```python
from build123d import *

# Parameters (mm, degrees)
SKETCH1_R           = 2
SKETCH1_R_2         = 2.7
SKETCH1_R_3         = 6.5
BOSS_EXTRUDE1_DEPTH = 2
SKETCH1_3_R         = 4.5
SKETCH1_3_R_2       = 3.5
SKETCH1_3_R_3       = 2
BOSS_EXTRUDE2_DEPTH = 26
CUT_EXTRUDE1_START  = -26
SKETCH1_4_R         = 4.5
SKETCH1_4_R_2       = 3.5
CUT_EXTRUDE1_DEPTH  = 5


with BuildPart() as part:
    # Sketch1 → Boss-Extrude1 (new body)
    with BuildSketch(Plane(origin=(0, 0, 0), x_dir=(1, 0, 0), z_dir=(0, 1, 0))):
        with BuildLine():
            ThreePointArc((31.3004561, 13.531128848), (24.112341238, 24.112341238), (13.531128848, 31.3004561))
            ThreePointArc((13.531128848, 31.3004561), (8.415102647, 35.598496025), (6.5, 42))
            ThreePointArc((6.5, 42), (0, 48.5), (-6.5, 42))
            ThreePointArc((-6.5, 42), (-8.415102647, 35.598496025), (-13.531128848, 31.3004561))
            ThreePointArc((-13.531128848, 31.3004561), (-24.112341238, 24.112341238), (-31.3004561, 13.531128848))
            ThreePointArc((-31.3004561, 13.531128848), (-35.598496025, 8.415102647), (-42, 6.5))
            ThreePointArc((-42, 6.5), (-48.5, 0), (-42, -6.5))
            ThreePointArc((-42, -6.5), (-35.598496025, -8.415102647), (-31.3004561, -13.531128848))
            ThreePointArc((-31.3004561, -13.531128848), (-24.112341238, -24.112341238), (-13.531128848, -31.3004561))
            ThreePointArc((-13.531128848, -31.3004561), (-8.415102647, -35.598496025), (-6.5, -42))
            ThreePointArc((-6.5, -42), (0, -48.5), (6.5, -42))
            ThreePointArc((6.5, -42), (8.415102647, -35.598496025), (13.531128848, -31.3004561))
            ThreePointArc((13.531128848, -31.3004561), (24.112341238, -24.112341238), (31.3004561, -13.531128848))
            ThreePointArc((31.3004561, -13.531128848), (35.598496025, -8.415102647), (42, -6.5))
            ThreePointArc((42, -6.5), (48.5, 0), (42, 6.5))
            ThreePointArc((42, 6.5), (35.598496025, 8.415102647), (31.3004561, 13.531128848))
        make_face()
        with Locations(Location((-42, 0, 0), (0, 0, 270))):
            Circle(SKETCH1_R, mode=Mode.SUBTRACT)
        with Locations(Location((-1.872696433, -20.916333524, 0), (0, 0, 270))):
            Circle(SKETCH1_R_2, mode=Mode.SUBTRACT)
        with Locations(Location((0, -42, 0), (0, 0, 270))):
            Circle(SKETCH1_R, mode=Mode.SUBTRACT)
        with Locations(Location((0, 0, 0), (0, 0, 270))):
            Circle(SKETCH1_R_3, mode=Mode.SUBTRACT)
        with Locations(Location((42, 0, 0), (0, 0, 270))):
            Circle(SKETCH1_R, mode=Mode.SUBTRACT)
        with Locations(Location((-17.177727969, 12.079969447, 0), (0, 0, 270))):
            Circle(SKETCH1_R_2, mode=Mode.SUBTRACT)
        with Locations(Location((19.050424402, 8.836364077, 0), (0, 0, 270))):
            Circle(SKETCH1_R_2, mode=Mode.SUBTRACT)
        with Locations(Location((0, 42, 0), (0, 0, 270))):
            Circle(SKETCH1_R, mode=Mode.SUBTRACT)
    extrude(amount=BOSS_EXTRUDE1_DEPTH)

    # Sketch1<3> → Boss-Extrude2 (add)
    with BuildSketch(Plane(origin=(0, 0, 0), x_dir=(1, 0, 0), z_dir=(0, 1, 0))):
        with BuildLine():
            ThreePointArc((46.5, 0), (42, 4.5), (37.5, 0))
            Line((37.5, 0), (38.5, 0))
            ThreePointArc((38.5, 0), (42, 3.5), (45.5, 0))
            Line((45.5, 0), (46.5, 0))
        make_face()
        with BuildLine():
            Line((38.5, 0), (37.5, 0))
            ThreePointArc((37.5, 0), (42, -4.5), (46.5, 0))
            Line((46.5, 0), (45.5, 0))
            ThreePointArc((45.5, 0), (42, -3.5), (38.5, 0))
        make_face()
        with BuildLine():
            ThreePointArc((45.5, 0), (42, 3.5), (38.5, 0))
            Line((38.5, 0), (40, 0))
            ThreePointArc((40, 0), (42, 2), (44, 0))
            Line((44, 0), (45.5, 0))
        make_face()
        with BuildLine():
            Line((40, 0), (38.5, 0))
            ThreePointArc((38.5, 0), (42, -3.5), (45.5, 0))
            Line((45.5, 0), (44, 0))
            ThreePointArc((44, 0), (42, -2), (40, 0))
        make_face()
        with Locations(Location((0, -42, 0), (0, 0, 270))):
            Circle(SKETCH1_3_R)
        with Locations((0, -42)):
            Circle(SKETCH1_3_R_2, mode=Mode.SUBTRACT)
        with Locations((0, -42)):
            Circle(SKETCH1_3_R_2)
        with Locations(Location((0, -42, 0), (0, 0, 270))):
            Circle(SKETCH1_3_R_3, mode=Mode.SUBTRACT)
        with Locations(Location((-42, 0, 0), (0, 0, 270))):
            Circle(SKETCH1_3_R)
        with Locations((-42, 0)):
            Circle(SKETCH1_3_R_2, mode=Mode.SUBTRACT)
        with Locations((-42, 0)):
            Circle(SKETCH1_3_R_2)
        with Locations(Location((-42, 0, 0), (0, 0, 270))):
            Circle(SKETCH1_3_R_3, mode=Mode.SUBTRACT)
        with Locations(Location((0, 42, 0), (0, 0, 270))):
            Circle(SKETCH1_3_R)
        with Locations((0, 42)):
            Circle(SKETCH1_3_R_2, mode=Mode.SUBTRACT)
        with Locations((0, 42)):
            Circle(SKETCH1_3_R_2)
        with Locations(Location((0, 42, 0), (0, 0, 270))):
            Circle(SKETCH1_3_R_3, mode=Mode.SUBTRACT)
    extrude(amount=-BOSS_EXTRUDE2_DEPTH)

    # Sketch1<4> → Cut-Extrude1 (cut)
    with BuildSketch(Plane(origin=(0, 0, 0), x_dir=(1, 0, 0), z_dir=(0, 1, 0)).offset(CUT_EXTRUDE1_START)):
        with Locations(Location((0, -42, 0), (0, 0, 270))):
            Circle(SKETCH1_4_R)
        with Locations(Location((0, -42, 0), (0, 0, 270))):
            Circle(SKETCH1_4_R_2, mode=Mode.SUBTRACT)
        with BuildLine():
            ThreePointArc((46.5, 0), (42, 4.5), (37.5, 0))
            Line((37.5, 0), (38.5, 0))
            ThreePointArc((38.5, 0), (42, 3.5), (45.5, 0))
            Line((45.5, 0), (46.5, 0))
        make_face()
        with BuildLine():
            Line((38.5, 0), (37.5, 0))
            ThreePointArc((37.5, 0), (42, -4.5), (46.5, 0))
            Line((46.5, 0), (45.5, 0))
            ThreePointArc((45.5, 0), (42, -3.5), (38.5, 0))
        make_face()
        with Locations(Location((0, 42, 0), (0, 0, 270))):
            Circle(SKETCH1_4_R)
        with Locations(Location((0, 42, 0), (0, 0, 270))):
            Circle(SKETCH1_4_R_2, mode=Mode.SUBTRACT)
        with Locations(Location((-42, 0, 0), (0, 0, 270))):
            Circle(SKETCH1_4_R)
        with Locations(Location((-42, 0, 0), (0, 0, 270))):
            Circle(SKETCH1_4_R_2, mode=Mode.SUBTRACT)
    extrude(amount=CUT_EXTRUDE1_DEPTH, mode=Mode.SUBTRACT)


solid = part.part
```
The listing builds one solid part. Answer for the finished solid, in the listing's coordinates (mm). A direction names the side the tool comes from. Coordinates: 2 decimals unless noted, no trailing zeros. Loops run counter-clockwise (first coordinate to the right, second up) from the corner with the lowest first, then second, coordinate; pieces in that order, holes last. Notation, with made-up numbers: (-7, -13.75) -> (24, -13.75) arc R27 cw to (24, 25.25) -> close; hole circle Ø3 at (40.25, 65.25). An arc over 180 degrees is marked (long way). Return JSON: item names as keys, results as strings. Group by question number.
(1) Find the intervals of material crossed by probe 1 along X at (y, z) = (-9.25, 42); probe 2 along X at (y, z) = (-12.75, -0.5); probe 3 along Y at (x, z) = (6.5, 32.5), in increasing order. Write a range as from..to.
(2) A cutting plane is placed at D-D on z = -18. Write down the section's boundary in (x, y), and give its area (3 significant figures).
(3) Which of the six approach directions +Z, -Z, +X, -X, +Y, -Y give full straight-line access (tool end or side, diameter ignored) to faces 5 (the cylindrical face through (0.1, 1, -48.5)), 6 (the flat face through (-4, -21, 42))?
(4) A cutting plane is placed at B-B on z = 0. Count the separate pieces of the cut face and the enclosed holes in it, and give its area (3 significant figures).
(5) A cutting plane is placed at C-C on x = -28. Write down the section's boundary in (y, z).
(6) Given pin 1 Ø4.5 at (x, z) = (-1.5, 41) entering from -Y; pin 2 Ø12 at (x, z) = (13.5, 8) entering from -Y, each flat-ended and moving along its own axis, determine where each tip first touches the part or whether it passes through.
(7) A cutting plane is placed at A-A on y = -12.5. Write down the section's boundary in (x, z).
(8) Determine the mould class of faces 1 (the flat face through (-2, -26, 44)), 2 (the cylindrical face through (0, -12, 40)), 3 (the cylindrical face through (0.154, -23.535, -45.497)), 4 (the cylindrical face through (-8.468, 0.986, 35.519)) for opening direction Z: released by +Z, released by -Z, zero draft, split by the parting line, or undercut.
The answers:
{
 "1": {"probe 1": "x = -4.5..-2, 2..4.5", "probe 2": "x = -46.47..-43.94, -40.06..-37.53, 37.53..40.06, 43.94..46.47", "probe 3": "y = 0..2"},
 "2": {"outline": "(-28.96, 0) -> (28.96, 0) -> (28.96, 2) -> (-28.96, 2) -> close", "area": "116 mm^2"},
 "3": {"face 5": "-Z, +Y, -Y", "face 6": "-Y"},
 "4": {"separate pieces": "4", "enclosed holes": "0", "area": "392 mm^2"},
 "5": {"outline": "(0, -19.46) -> (2, -19.46) -> (2, 19.46) -> (0, 19.46) -> close"},
 "6": {"pin 1": "stops at y = -26", "pin 2": "stops at y = 0"},
 "7": {"outline": "circle Ø9 at (-42, 0); circle Ø9 at (0, -42); circle Ø9 at (0, 42); circle Ø9 at (42, 0); hole circle Ø4 at (-42, 0); hole circle Ø4 at (0, -42); hole circle Ø4 at (0, 42); hole circle Ø4 at (42, 0)"},
 "8": {"face 1": "zero draft", "face 2": "undercut", "face 3": "undercut", "face 4": "released by +Z"}
}
